Part model, mm, in its own coordinate system. Face numbers are marked on the shaded views. Give positions to 0.01 mm unless a question says otherwise; leave off trailing zeros. Write each loop counter-clockwise with the first axis right and the second up, starting at its lowest first coordinate (ties: lowest second). Pieces come first, ordered by that corner, then holes.
```python
from build123d import *

# Parameters (mm, degrees)
F0_R     = 5
F1_DEPTH = 1
F3_DEPTH = 5
F4_R     = 2.25
F5_DEPTH = 3.5
F6_R     = 1
F7_DEPTH = 25
F8_R     = 2


with BuildPart() as f1:
    # F0 (on Front) → F1 (new body)
    with BuildSketch(Plane.XZ):
        Circle(F0_R)
    extrude(amount=F1_DEPTH)

    # F2 (on face) → F3 (join)
    with BuildSketch(Plane.XZ.offset(1)):
        with BuildLine():
            ThreePointArc((-1, 25), (-4.551972, 12.723625), (-5.75, 0))
            ThreePointArc((-5.75, 0), (0, -5.75), (5.75, 0))
            ThreePointArc((5.75, 0), (4.551972, 12.723625), (1, 25))
            Line((1, 25), (-1, 25))
        make_face()
    extrude(amount=F3_DEPTH)

    # F4 (on face) → F5 (cut)
    with BuildSketch(Plane(origin=(0, 0, 0), x_dir=(-1, 0, 0), z_dir=(0, 1, 0))):
        Circle(F4_R)
    extrude(amount=-F5_DEPTH, mode=Mode.SUBTRACT)

    # F6 (on face) → F7 (cut)
    with BuildSketch(Plane.XZ.offset(6)):
        Circle(F6_R)
    extrude(amount=-F7_DEPTH, mode=Mode.SUBTRACT)

    # F8
    f8_edges = [f1.edges().sort_by_distance(p)[0] for p in [
        (-1, -3.5, 25),
    ]]
    fillet(f8_edges, radius=F8_R)


solid = f1.part
```
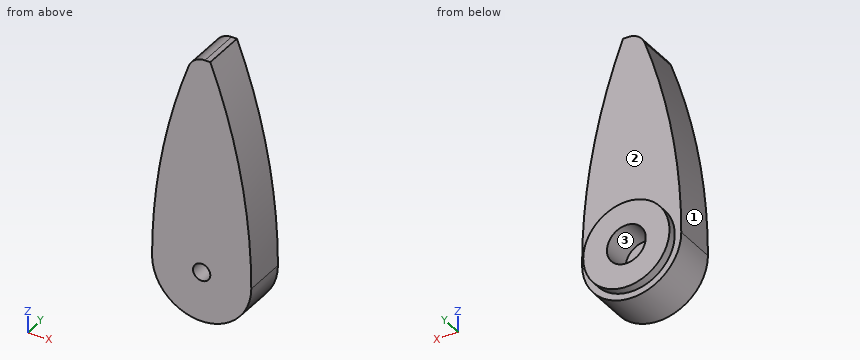
1) Saw through at B-B, the plane y = -1.9. Write the cut outline in (x, z).
Answers follow:
outline: (-5.75, 0) arc R5.75 ccw to (5.75, 0) arc R68.16 ccw to (1, 25) - (0.38, 25) arc R2 ccw to (-1.5, 23.7) arc R68.16 ccw to start; hole circle Ø4.5 at (0, 0)
2) Saw through at C-C, the plane x = -4. Write the cut outline in (y, z).
Answers follow:
outline: (-6, -4.13) - (-1, -4.13) - (-1, -3) - (0, -3) - (0, 3) - (-1, 3) - (-1, 15.35) - (-6, 15.35) - close
3) Wall check: L1, parallel to Y at x = 4.5, z = 12.5; L2, parallel to Y at x = 0.5, z = -2; L3, parallel to Z at x = 0, y = -2.7. Give the ranges that are in metal, low to high.
Answers follow:
L1: y = -6 to -1
L2: y = -6 to -3.5
L3: z = -5.75 to -2.25, 2.25 to 24.96
4) Saw through at A-A, the plane x = -0.5. Write the cut outline in (y, z).
Answers follow:
outline: (-6, -5.73) - (-1, -5.73) - (-1, -4.97) - (0, -4.97) - (0, -2.19) - (-3.5, -2.19) - (-3.5, -0.87) - (-6, -0.87) - close; (-6, 0.87) - (-3.5, 0.87) - (-3.5, 2.19) - (0, 2.19) - (0, 4.97) - (-1, 4.97) - (-1, 24.8) - (-6, 24.8) - close
5) Pin check, flat tips, straight feed: pin 1 Ø5 at (x, z) = (1, 0.5) entering from +Y; pin 2 Ø2 at (y, z) = (-1.5, 6) entering from -X; pin 3 Ø3 at (y, z) = (-3.5, 21) entering from +X; pin 4 Ø1.6 at (x, z) = (0, 0) entering from +Y. Stop position of each tip, or through.
Answers follow:
pin 1: stops at y = 0
pin 2: stops at x = -5.57
pin 3: stops at x = 2.9
pin 4: passes through
6) Two-plate mould, pull along Z, no slides. Class the marked faces 1, 2 and 3: +Z half, -Z half, draft (parallel to the pull), parting line (faces both ways), or undercut.
Answers follow:
face 1: +Z half
face 2: draft
face 3: undercut
7) Saw through at D-D, the plane y = -4.1. Write the cut outline in (x, z), then the cut area to 3 significant figures.
Answers follow:
outline: (-5.75, 0) arc R5.75 ccw to (5.75, 0) arc R68.16 ccw to (1, 25) - (0.38, 25) arc R2 ccw to (-1.5, 23.7) arc R68.16 ccw to start; hole circle Ø2 at (0, 0)
area: 258 mm2
